from build123d import *

# Parameters (mm, degrees)
EXTRUDE_1_DEPTH     = 30.48
SKETCH_4_R          = 3.302
EXTRUDE_2_DEPTH     = 6.12463
SKETCH_5_W          = 82.55
SKETCH_5_H          = 48.620400001
EXTRUDE_3_DEPTH     = 3
SKETCH_6_R          = 1.5
CUT_EXTRUDE_1_DEPTH = 3
SKETCH_7_R          = 1.5
CUT_EXTRUDE_2_DEPTH = 2
SKETCH_8_R          = 1.5
CUT_EXTRUDE_3_DEPTH = 10
SKETCH_9_W          = 8.255
SKETCH_9_H          = 5
CUT_EXTRUDE_4_DEPTH = 19


with BuildPart() as part:
    # 스케치3 → 보스-돌출1 (new body)
    with BuildSketch(Plane.XY):
        Polygon((21517.522317655, 8422.852866974), (21525.777317655, 8422.852866974), (21525.777317655, 8382.487466973), (21591.817317655, 8382.487466973), (21591.817317655, 8422.852866974), (21600.072317655, 8422.852866974), (21600.072317655, 8374.232466973), (21517.522317655, 8374.232466973), align=None)
    extrude(amount=EXTRUDE_1_DEPTH)

    # 스케치4 → 보스-돌출2 (add)
    with BuildSketch(Plane(origin=(0, 8374.232466973, 0), x_dir=(-1, 0, 0), z_dir=(0, -1, 0))):
        with Locations((-21576.717457655, -15.24)):
            Circle(SKETCH_4_R)
    extrude(amount=EXTRUDE_2_DEPTH)

    # 스케치5 → 보스-돌출3 (add)
    with BuildSketch(Plane(origin=(0, 0, 0), x_dir=(-1, 0, 0), z_dir=(0, 0, -1))):
        with Locations((-21558.797317655, 8398.542666974)):
            Rectangle(SKETCH_5_W, SKETCH_5_H)
    extrude(amount=EXTRUDE_3_DEPTH)

    # 스케치6 → 컷-돌출1 (cut)
    with BuildSketch(Plane.XY):
        with Locations((21577.97657564, 8407.672466973)):
            Circle(SKETCH_6_R)
        with Locations((21567.97657564, 8407.672466973)):
            Circle(SKETCH_6_R)
        with Locations((21567.97657564, 8397.672466973)):
            Circle(SKETCH_6_R)
        with Locations((21577.97657564, 8397.672466973)):
            Circle(SKETCH_6_R)
    extrude(amount=-CUT_EXTRUDE_1_DEPTH, mode=Mode.SUBTRACT)

    # 스케치7 → 컷-돌출2 (cut)
    with BuildSketch(Plane.XY):
        Polygon((21569.593155483, 8410.472467064), (21566.359995798, 8410.472467064), (21564.743415955, 8407.672466973), (21566.359995798, 8404.872466883), (21569.593155483, 8404.872466883), (21571.209735325, 8407.672466973), align=None)
        with Locations((21567.97657564, 8407.672466973)):
            Circle(SKETCH_7_R, mode=Mode.SUBTRACT)
        Polygon((21569.593155483, 8400.472467064), (21566.359995798, 8400.472467064), (21564.743415955, 8397.672466973), (21566.359995798, 8394.872466883), (21569.593155483, 8394.872466883), (21571.209735325, 8397.672466973), align=None)
        with Locations((21567.97657564, 8397.672466973)):
            Circle(SKETCH_7_R, mode=Mode.SUBTRACT)
        Polygon((21579.593155483, 8400.472467064), (21576.359995798, 8400.472467064), (21574.743415955, 8397.672466973), (21576.359995798, 8394.872466883), (21579.593155483, 8394.872466883), (21581.209735325, 8397.672466973), align=None)
        with Locations((21577.97657564, 8397.672466973)):
            Circle(SKETCH_7_R, mode=Mode.SUBTRACT)
        Polygon((21579.593155483, 8410.472467064), (21576.359995798, 8410.472467064), (21574.743415955, 8407.672466973), (21576.359995798, 8404.872466883), (21579.593155483, 8404.872466883), (21581.209735325, 8407.672466973), align=None)
        with Locations((21577.97657564, 8407.672466973)):
            Circle(SKETCH_7_R, mode=Mode.SUBTRACT)
    extrude(amount=-CUT_EXTRUDE_2_DEPTH, mode=Mode.SUBTRACT)

    # 스케치8 → 컷-돌출3 (cut)
    with BuildSketch(Plane(origin=(0, 8422.852866974, 0), x_dir=(1, 0, 0), z_dir=(0, 1, 0))):
        with Locations((21597.072317655, -6)):
            Circle(SKETCH_8_R)
        with Locations((21597.072317655, -24.48)):
            Circle(SKETCH_8_R)
        with Locations((21520.522317655, -24.48)):
            Circle(SKETCH_8_R)
        with Locations((21520.522317655, -6)):
            Circle(SKETCH_8_R)
    extrude(amount=-CUT_EXTRUDE_3_DEPTH, mode=Mode.SUBTRACT)

    # 스케치9 → 컷-돌출4 (cut)
    with BuildSketch(Plane.XY.offset(30.48)):
        with Locations((21595.944817655, 8388.987466973)):
            Rectangle(SKETCH_9_W, SKETCH_9_H)
    extrude(amount=-CUT_EXTRUDE_4_DEPTH, mode=Mode.SUBTRACT)


solid = part.part
Source: CAD feature listing. Evaluate the final solid. Frame: model axes, mm. A direction names the side the tool comes from. Give positions to 0.01 mm unless a question says otherwise; leave off trailing zeros. Write each loop counter-clockwise with the first axis right and the second up, starting at its lowest first coordinate (ties: lowest second). Pieces come first, ordered by that corner, then holes. Notation, with made-up numbers: M 54.5,17 L 104.5,17 A24 cw 104.5,53 Z; hole C 45.25,86.25 d10. An arc over 180 degrees is marked long. Answer as a JSON object with one key per item and string values.
Q1. Cut plane C-C, the plane z = 6. Return the cut outline in (x, y), then the cut area to 3 significant figures.
Geometry check:
{"outline": "M 21517.52,8374.23 L 21600.07,8374.23 L 21600.07,8422.85 L 21598.57,8422.85 L 21598.57,8412.85 L 21595.57,8412.85 L 21595.57,8422.85 L 21591.82,8422.85 L 21591.82,8382.49 L 21525.78,8382.49 L 21525.78,8422.85 L 21522.02,8422.85 L 21522.02,8412.85 L 21519.02,8412.85 L 21519.02,8422.85 L 21517.52,8422.85 Z", "area": "1,290 mm^2"}
Q2. Mould query, pull axis X, two halves, no side actions, for faces 4 (the face through (21550, 8382, 30.48)), 5 (the face through (21570.413, 8399.053, -0.986)). Classes: +X half, -X half, draft (parallel to the pull), parting line (faces both ways), or undercut.
Geometry check:
{"face 4": "draft", "face 5": "undercut"}
Q3. Cut plane A-A, the plane z = 24.48. Return the cut outline in (x, y).
Geometry check:
{"outline": "M 21517.52,8374.23 L 21600.07,8374.23 L 21600.07,8386.49 L 21591.82,8386.49 L 21591.82,8382.49 L 21525.78,8382.49 L 21525.78,8422.85 L 21522.02,8422.85 L 21522.02,8412.85 L 21519.02,8412.85 L 21519.02,8422.85 L 21517.52,8422.85 Z; M 21591.82,8391.49 L 21600.07,8391.49 L 21600.07,8422.85 L 21598.57,8422.85 L 21598.57,8412.85 L 21595.57,8412.85 L 21595.57,8422.85 L 21591.82,8422.85 Z"}
Q4. Contact query for flat-ended pins moving along their axis: P1, Ø20, axis at x = 21574.5, y = 8393, coming from the +Z side; P2, Ø2.5, axis at x = 21577.98, y = 8397.67, coming from the -Z side; P3, Ø1.7, axis at x = 21579.5, y = 8407.5, coming from the +Z side; P4, Ø15, axis at x = 21575, z = 17, coming from the +Y side. Output: stop coordinate, or through.
Geometry check:
{"P1": "stops at z = 0", "P2": "passes through", "P3": "stops at z = -2", "P4": "stops at y = 8382.49"}
Q5. Cut plane B-B, the plane y = 8393.5. Return the cut outline in (x, z).
Geometry check:
{"outline": "M 21517.52,-3 L 21600.07,-3 L 21600.07,30.48 L 21591.82,30.48 L 21591.82,0 L 21525.78,0 L 21525.78,30.48 L 21517.52,30.48 Z"}
Q6. Cut plane D-D, the plane x = 21537. Return the cut outline in (y, z).
Geometry check:
{"outline": "M 8374.23,-3 L 8422.85,-3 L 8422.85,0 L 8382.49,0 L 8382.49,30.48 L 8374.23,30.48 Z"}
Q7. Access query for faces 1 (the face through (21568, 8410.472, -1)), 2 (the face through (21521, 8412.853, 24)), 3 (the face through (21596, 8391.487, 21)). Directions: +Z, -Z, +X, -X, +Y, -Y. A direction counts if a zero-diameter tool reaches every point of the face in a straight line with its end or side. Return the directions, or none.
Geometry check:
{"face 1": "+Z", "face 2": "+Y", "face 3": "+Z, +X"}
Q8. Ray query, line 1 along X through (y, z) = (8417, 6); line 2 along X through (y, z) = (8392, 3); line 3 along Y through (x, z) = (21576, 3.5). Return the intervals inside material, ascending.
Geometry check:
{"line 1": "x = 21517.52 to 21519.02, 21522.02 to 21525.78, 21591.82 to 21595.57, 21598.57 to 21600.07", "line 2": "x = 21517.52 to 21525.78, 21591.82 to 21600.07", "line 3": "y = 8374.23 to 8382.49"}
